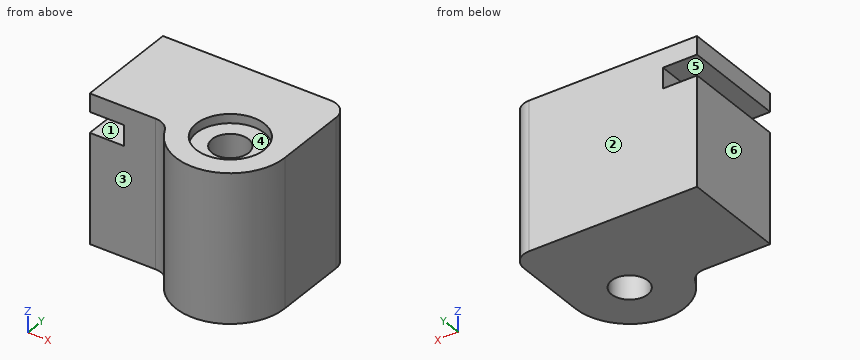
from build123d import *

# Parameters (mm, degrees)
SKETCH028_R     = 1.6
PAD016_DEPTH    = 13
SKETCH029_W     = 3
SKETCH029_H     = 1.8
POCKET010_DEPTH = 12.861
SKETCH030_R     = 3
POCKET011_DEPTH = 0.8


with BuildPart() as part:
    # Sketch028 (on Face1 of Binder006) → Pad016 (new body)
    with BuildSketch(Plane.XY.offset(95.6)):
        with BuildLine():
            ThreePointArc((38.842146, -4.595), (44.233162, -7.223038), (47.98, -2.54))
            Line((47.98, 3.92), (47.98, -2.54))
            ThreePointArc((47.98, 3.92), (47.511371, 5.051371), (46.38, 5.52))
            Line((31.61, 5.52), (46.38, 5.52))
            Line((31.61, -3.68), (31.61, 5.52))
            Line((37.396195, -3.68), (31.61, -3.68))
            ThreePointArc((38.842146, -4.595), (38.251765, -3.927964), (37.396195, -3.68))
        make_face()
        with Locations((43.18, -2.54)):
            Circle(SKETCH028_R, mode=Mode.SUBTRACT)
    extrude(amount=PAD016_DEPTH)

    # Sketch029 (on Face4 of Pad016) → Pocket010 (cut, through all)
    with BuildSketch(Plane(origin=(0, 5.52, 0), x_dir=(-1, 0, 0), z_dir=(0, 1, 0))):
        with Locations((-33.11, 106.1)):
            Rectangle(SKETCH029_W, SKETCH029_H)
    extrude(amount=-POCKET010_DEPTH, mode=Mode.SUBTRACT)

    # Sketch030 (on Face5 of Pocket010) → Pocket011 (cut)
    with BuildSketch(Plane.XY.offset(108.6)):
        with Locations((43.18, -2.54)):
            Circle(SKETCH030_R)
    extrude(amount=-POCKET011_DEPTH, mode=Mode.SUBTRACT)


solid = part.part
Design review of the part built by this model. Coordinates are the model's own, in mm. Face numbers are marked on the shaded views. A direction names the side the tool comes from. Give positions to 0.01 mm unless a question says otherwise; leave off trailing zeros. Loops run counter-clockwise (first coordinate to the right, second up) from the corner with the lowest first, then second, coordinate; pieces in that order, holes last. Notation, with made-up numbers: M 56,48.5 L 95,48.5 A28 cw 95,76.5 Z; hole C 84.5,-27.5 d1. An arc over 180 degrees is marked long. Write item = value, one per line.
Q1. We need section B-B (x = 43.18). Give the boundary of the cut face in (y, z).
Output values:
outline = M -7.34,95.6 L -4.14,95.6 L -4.14,107.8 L -5.54,107.8 L -5.54,108.6 L -7.34,108.6 Z; M -0.94,95.6 L 5.52,95.6 L 5.52,108.6 L 0.46,108.6 L 0.46,107.8 L -0.94,107.8 Z
Q2. We need section C-C (y = -1.25). Give the boundary of the cut face in (x, z).
Output values:
outline = M 31.61,95.6 L 42.23,95.6 L 42.23,107.8 L 40.47,107.8 L 40.47,108.6 L 31.61,108.6 L 31.61,107 L 34.61,107 L 34.61,105.2 L 31.61,105.2 Z; M 44.13,95.6 L 47.98,95.6 L 47.98,108.6 L 45.89,108.6 L 45.89,107.8 L 44.13,107.8 Z
Q3. To check wall thickness, follow line 1 (X direction, y = -2.54, z = 100); line 2 (Z direction, x = 32.75, y = 0.25); line 3 (Y direction, x = 43.18, z = 100.5). State the ranges of each line that lie inside material, in increasing order. Write a range as [from, to].
Output values:
line_1 = [31.61, 41.58], [44.78, 47.98]
line_2 = [95.6, 105.2], [107, 108.6]
line_3 = [-7.34, -4.14], [-0.94, 5.52]
Q4. For the marked faces 1, 2 and 3, list the 3-axis set-ups (+Z, -Z, +X, -X, +Y, -Y) from which the entire face can be reached by the end or side of a thin tool; tool diameter is ignored.
Output values:
face_1 = -X, +Y, -Y
face_2 = +Z, -Z, +X, -X, +Y
face_3 = +Z, -Z, -X, -Y
Q5. Insertion check: pin 1 (1.7 mm diameter, centred on x = 33.5, z = 103.5, fed in from -Y); pin 2 (1.8 mm diameter, centred on x = 44.5, y = -4, fed in from +Z). Each pin has a flat end and moves straight along its axis. Give the tip position at first contact, or say it passes through.
Output values:
pin_1 = -3.68
pin_2 = 107.8
Q6. We need section D-D (y = 1.5). Give the boundary of the cut face in (x, z), plus the area to 3 significant figures.
Output values:
outline = M 31.61,95.6 L 47.98,95.6 L 47.98,108.6 L 31.61,108.6 L 31.61,107 L 34.61,107 L 34.61,105.2 L 31.61,105.2 Z
area = 207 mm^2
Q7. We need section A-A (z = 104.5). Give the boundary of the cut face in (x, y) (3 decimals), plus the area to 3 significant figures.
Output values:
outline = M 31.61,-3.68 L 37.396,-3.68 A1.6 cw 38.842,-4.595 A4.8 ccw 47.98,-2.54 L 47.98,3.92 A1.6 ccw 46.38,5.52 L 31.61,5.52 Z; hole C 43.18,-2.54 d3.2
area = 168 mm^2
Q8. Draft analysis for pull direction X (two halves, no side actions). For the marked faces 4, 5 and 6, state which applies: +X half, -X half, draft (parallel to the pull), parting line (faces both ways), or undercut.
Output values:
face_4 = undercut
face_5 = draft
face_6 = -X half
